CAD build for the part. Positions are in the model's coordinates, mm. Face numbers are marked on the shaded views. Coordinates: 2 decimals unless noted, no trailing zeros. Loops run counter-clockwise (first coordinate to the right, second up) from the corner with the lowest first, then second, coordinate; pieces in that order, holes last. Notation, with made-up numbers: (0, 58) -> (46, 58) arc R17 ccw to (46, 70) -> close; hole circle Ø9 at (75.25, -7). An arc over 180 degrees is marked (long way). Write item = value, one per line. Start each with the question number.
(1) Flat gauge pins, fed straight in: P1, Ø12, axis at x = 316.5, z = 10.5, coming from the -Y side; P2, Ø1.8, axis at y = 38, z = 31, coming from the +X side; P3, Ø4, axis at x = 298.5, y = 10, coming from the -Z side; P4, Ø0.9, axis at y = -1.5, z = -8.5, coming from the +X side. Where does each tip first touch, or does it go through?
(2) Band-saw the part on C-C (x = 109). Write the cut outline in (y, z), and give its area (3 significant figures).
(3) Pull direction X, two halves, no side cores. Call the marked faces 1 and 2: +X half, -X half, draft (parallel to the pull), parting line (faces both ways), or undercut.
(4) Band-saw the part on A-A (x = 37). Write the cut outline in (y, z).
(5) Band-saw the part on D-D (z = 15). Write the cut outline in (x, y).
(6) Band-saw the part on B-B (y = 22). Write the cut outline in (x, z).
(7) Drill centre lines: line 1 (X direction, y = 26, z = -12); line 2 (Y direction, x = 20, z = 5.5); line 3 (Z direction, x = 70, y = 6). Where is each one in solid material? Low to high. Write a range as from..to.
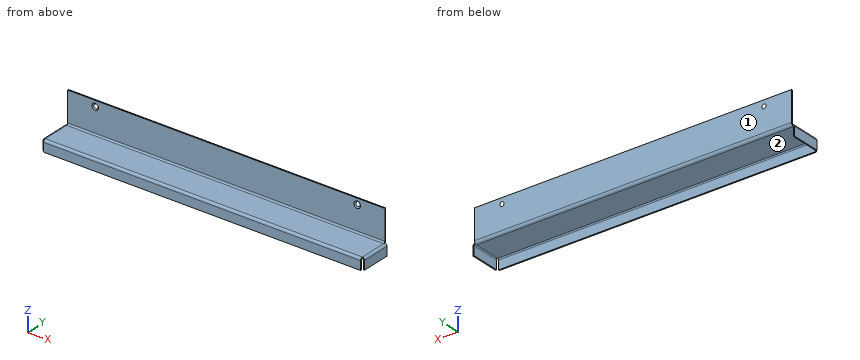
```python
from build123d import *

# Parameters (mm, degrees)
SKETCH_1_W                       = 426
SKETCH_1_H                       = 39.2
SM_BASE_FLANGE_1_DEPTH           = 1.5
SM_EDGE_FLANGE_2_DEPTH           = 39.2
SM_EDGE_FLANGE_3_DEPTH           = 426
SM_EDGE_FLANGE_4_DEPTH           = 39.2
SM_EDGE_FLANGE_5_STRIP_W         = 10
SM_EDGE_FLANGE_5_STRIP_H         = 1.5
SM_EDGE_FLANGE_5_STRIP_CUT_DEPTH = 426
SM_EDGE_FLANGE_5_DEPTH           = 426
SKETCH_28_R                      = 2.3
CUT_EXTRUDE_1_DEPTH              = 434.111810044
CHAMFER_1_SIZE                   = 2.05


# Sheet-metal steps are written as plain solids
with BuildPart() as part:
    # Sketch 1 → Базовая кромка1 (new body)
    with BuildSketch(Plane.XY):
        with Locations((213, 19.6)):
            Rectangle(SKETCH_1_W, SKETCH_1_H)
    extrude(amount=-SM_BASE_FLANGE_1_DEPTH)

    # Ребро-кромка2 section (across the edge) → Ребро-кромка2 (add)
    with BuildSketch(Plane(origin=(-1.5, 0, -1.5), x_dir=(1, 0, 0), z_dir=(0, 1, 0))):
        with BuildLine():
            Line((-1.5, 1.5), (-1.5, 13.5))
            Line((-1.5, 13.5), (0, 13.5))
            Line((0, 13.5), (0, 1.5))
            ThreePointArc((0, 1.5), (0.439339828, 0.439339828), (1.5, 0))
            Line((1.5, 0), (1.5, -1.5))
            ThreePointArc((1.5, -1.5), (-0.621320344, -0.621320344), (-1.5, 1.5))
        make_face()
    extrude(amount=SM_EDGE_FLANGE_2_DEPTH)

    # Ребро-кромка3 section (across the edge) → Ребро-кромка3 (add)
    with BuildSketch(Plane(origin=(426, -1.5, -1.5), x_dir=(0, 1, 0), z_dir=(-1, 0, 0))):
        with BuildLine():
            Line((-1.5, 1.5), (-1.5, 13.5))
            Line((-1.5, 13.5), (0, 13.5))
            Line((0, 13.5), (0, 1.5))
            ThreePointArc((0, 1.5), (0.439339828, 0.439339828), (1.5, 0))
            Line((1.5, 0), (1.5, -1.5))
            ThreePointArc((1.5, -1.5), (-0.621320344, -0.621320344), (-1.5, 1.5))
        make_face()
    extrude(amount=SM_EDGE_FLANGE_3_DEPTH)

    # Ребро-кромка4 section (across the edge) → Ребро-кромка4 (add)
    with BuildSketch(Plane(origin=(427.5, 39.2, -1.5), x_dir=(-1, 0, 0), z_dir=(0, -1, 0))):
        with BuildLine():
            Line((-1.5, 1.5), (-1.5, 13.5))
            Line((-1.5, 13.5), (0, 13.5))
            Line((0, 13.5), (0, 1.5))
            ThreePointArc((0, 1.5), (0.439339828, 0.439339828), (1.5, 0))
            Line((1.5, 0), (1.5, -1.5))
            ThreePointArc((1.5, -1.5), (-0.621320344, -0.621320344), (-1.5, 1.5))
        make_face()
    extrude(amount=SM_EDGE_FLANGE_4_DEPTH)

    # Ребро-кромка5 strip (across the edge) → Ребро-кромка5 strip cut (cut)
    with BuildSketch(Plane(origin=(426, 39.2, 0), x_dir=(0, -1, 0), z_dir=(-1, 0, 0))):
        with Locations((-3, -0.75)):
            Rectangle(SM_EDGE_FLANGE_5_STRIP_W, SM_EDGE_FLANGE_5_STRIP_H)
    extrude(amount=SM_EDGE_FLANGE_5_STRIP_CUT_DEPTH, mode=Mode.SUBTRACT)

    # Ребро-кромка5 section (across the edge) → Ребро-кромка5 (add)
    with BuildSketch(Plane(origin=(426, 39.2, 0), x_dir=(0, -1, 0), z_dir=(-1, 0, 0))):
        with BuildLine():
            Line((-1.5, 2), (-1.5, 42))
            Line((-1.5, 42), (0, 42))
            Line((0, 42), (0, 2))
            ThreePointArc((0, 2), (0.585786438, 0.585786438), (2, 0))
            Line((2, 0), (2, -1.5))
            ThreePointArc((2, -1.5), (-0.474873734, -0.474873734), (-1.5, 2))
        make_face()
    extrude(amount=SM_EDGE_FLANGE_5_DEPTH)

    # Эскиз28 → Вырез-Вытянуть1 (cut, through all)
    with BuildSketch(Plane.XZ.offset(-39.2)):
        with Locations(Location((37, 34, 0), (0, 0, 270))):
            Circle(SKETCH_28_R)
        with Locations(Location((389, 34, 0), (0, 0, 270))):
            Circle(SKETCH_28_R)
    extrude(amount=-CUT_EXTRUDE_1_DEPTH, mode=Mode.SUBTRACT)

    # Фаска1
    # the kernel refuses this chamfer: 2.05 mm, written as the material it takes off along each edge
    with BuildSketch(Plane(origin=(389, 39.2, 34), x_dir=(0, 0, -1), z_dir=(-1, 0, 0))) as chamfer_1_piece_1:
        Polygon((2.3 + CHAMFER_1_SIZE, 0), (2.3, -CHAMFER_1_SIZE), (2.3, 0), align=None)
    revolve(axis=Axis((389, 39.2, 34), (0, -1, 0)), mode=Mode.SUBTRACT)
    with BuildSketch(Plane(origin=(37, 39.2, 34), x_dir=(0, 0, -1), z_dir=(-1, 0, 0))) as chamfer_1_piece_2:
        Polygon((2.3 + CHAMFER_1_SIZE, 0), (2.3, -CHAMFER_1_SIZE), (2.3, 0), align=None)
    revolve(axis=Axis((37, 39.2, 34), (0, -1, 0)), mode=Mode.SUBTRACT)


solid = part.part
```
Findings below:
q1.P1 = 39.2
q1.P2 = through
q1.P3 = -1.5
q1.P4 = 426
q2.outline = (-3, -15) -> (-1.5, -15) -> (-1.5, -3) arc R1.5 cw to (0, -1.5) -> (37.2, -1.5) arc R3.5 ccw to (40.7, 2) -> (40.7, 42) -> (39.2, 42) -> (39.2, 2) arc R2 cw to (37.2, 0) -> (0, 0) arc R3 ccw to (-3, -3) -> close
q2.area = 146 mm²
q3.face_1 = draft
q3.face_2 = undercut
q4.outline = (-3, -15) -> (-1.5, -15) -> (-1.5, -3) arc R1.5 cw to (0, -1.5) -> (37.2, -1.5) arc R3.5 ccw to (40.7, 2) -> (40.7, 31.15) -> (39.2, 29.65) -> (39.2, 2) arc R2 cw to (37.2, 0) -> (0, 0) arc R3 ccw to (-3, -3) -> close; (39.2, 38.35) -> (40.7, 36.85) -> (40.7, 42) -> (39.2, 42) -> close
q5.outline = (0, 39.2) -> (426, 39.2) -> (426, 40.7) -> (0, 40.7) -> close
q6.outline = (-3, -15) -> (-1.5, -15) -> (-1.5, -3) arc R1.5 cw to (0, -1.5) -> (426, -1.5) arc R1.5 cw to (427.5, -3) -> (427.5, -15) -> (429, -15) -> (429, -3) arc R3 ccw to (426, 0) -> (0, 0) arc R3 ccw to (-3, -3) -> close
q7.line_1 = -3..-1.5, 427.5..429
q7.line_2 = 39.2..40.7
q7.line_3 = -1.5..0
